Check sheet for the modelled part. Datum: model origin and axes. Units: mm. A direction names the side the tool comes from. Give positions to 0.01 mm unless a question says otherwise; leave off trailing zeros. Order: outer loops, then holes, each group sorted by start corner. A loop starts at its lowest first (then second) coordinate and runs counter-clockwise, first axis right, second up.
```python
from build123d import *

# Parameters (mm, degrees)
ESBO_O2_R             = 3
CORTE_EXTRUS_O1_DEPTH = 3.6
CHANFRO2_SIZE         = 1.5
CHANFRO2_SIZE2        = 3.216760381
CHANFRO3_SIZE         = 1.5
FILETE3_R             = 0.5


with BuildPart() as part:
    # Esboço1 → Revolução1 (revolve)
    with BuildSketch(Plane.XY, mode=Mode.PRIVATE) as revolu_o1_sk:
        Polygon((0, 0), (71, 0), (71, 7), (61, 7), (61, 5.8), (58.5, 5.8), (58.5, 7), (30.5, 7), (30.5, 5), (0, 5), align=None)
    revolve(revolu_o1_sk.sketch.rotate(Axis((0, 0, 0), (1, 0, 0)), 90), axis=Axis((0, 0, 0), (1, 0, 0)))

    # Esboço2 → Corte-extrusão1 (cut)
    with BuildSketch(Plane.ZY):
        Circle(ESBO_O2_R)
    extrude(amount=-CORTE_EXTRUS_O1_DEPTH, mode=Mode.SUBTRACT)

    # Chanfro2
    chanfro2_edges = [part.edges().sort_by_distance(p)[0] for p in [
        (0, 0, -3),
    ]]
    chanfro2_side = [part.faces().sort_by_distance(p)[0] for p in [
        (0, 0, -4.858578644),
    ]]
    chamfer(chanfro2_edges, length=CHANFRO2_SIZE, length2=CHANFRO2_SIZE2, reference=chanfro2_side[0])

    # Chanfro3
    chanfro3_edges = [part.edges().sort_by_distance(p)[0] for p in [
        (30.5, 0, -7),
    ]]
    chamfer(chanfro3_edges, length=CHANFRO3_SIZE)

    # Filete3
    filete3_edges = [part.edges().sort_by_distance(p)[0] for p in [
        (71, 0, -7),
        (58.5, 0, -7),
        (61, 0, -7),
    ]]
    fillet(filete3_edges, radius=FILETE3_R)


solid = part.part
```
(1) Material ranges on L1, parallel to Y at x = 3.35, z = 0; L2, parallel to Z at x = 44, y = 0.25; L3, parallel to X at y = 2.75, z = 0, recorded low to high.
Response values:
L1: y = -5 to -3, 3 to 5
L2: z = -7 to 7
L3: x = 3.6 to 71
(2) Gauge pin test, flat ends, axial feed: pin 1 Ø3 at (x, y) = (28.5, 4.5) entering from -Z; pin 2 Ø6.5 at (y, z) = (-1, 0) entering from -X; pin 3 Ø1 at (x, z) = (8, -3.5) entering from -Y. Record the tip position at first contact, or that the pin passes through.
Response values:
pin 1: stops at z = -4
pin 2: stops at x = 0.54
pin 3: stops at y = -4
(3) Cross-section at D-D on x = 49. Enter the section's corners in (y, z).
Response values:
outline: circle Ø14 at (0, 0)
(4) Set-up check for faces 4 (the face through (65.94, 6.21, 3.23)), 5 (the face through (3.6, 0, 0)), 6 (the face through (61, 0, -6)): record each of +Z, -Z, +X, -X, +Y, -Y from which the full face is reachable in a straight line by a thin tool's end or side.
Response values:
face 4: +X, -X
face 5: -X
face 6: none
(5) Release check for a two-part mould opening along Y. For faces 1 (the face through (3.06, -1.87, -2.44)), 2 (the face through (58.5, 0, 6)), 3 (the face through (44.82, 6.21, 3.23)) record: released by +Y, released by -Y, zero draft, split by the parting line, or undercut.
Response values:
face 1: undercut
face 2: zero draft
face 3: split by the parting line
(6) Cross-section at C-C on x = 24. Enter the section's corners in (y, z).
Response values:
outline: circle Ø10 at (0, 0)
